```python
from build123d import *

# Parameters (mm, degrees)
F0_W     = 134.2057809234
F0_H     = 157.6057672501
F1_DEPTH = 25.4
F2_W     = 134.2057809234
F2_H     = 11.8888095021
F3_DEPTH = 50.8
F4_R     = 3.3067851736
F4_R_2   = 4.5017573087
F5_DEPTH = 25.4
F6_R     = 5.7930300282
F6_R_2   = 5.5883167401
F7_DEPTH = 25.4


with BuildPart() as f1:
    # F0 (on Front) → F1 (new body)
    with BuildSketch(Plane.XZ):
        with Locations((-1.6366653144, 9.6122771502)):
            Rectangle(F0_W, F0_H)
    extrude(amount=F1_DEPTH)

    # F2 (on face) → F3 (join)
    with BuildSketch(Plane.XZ.offset(25.4)):
        with Locations((-1.6366653144, -63.2462017238)):
            Rectangle(F2_W, F2_H)
    extrude(amount=F3_DEPTH)

    # F4 (on face) → F5 (cut)
    with BuildSketch(Plane.XY.offset(-57.3017969728)):
        with Locations((-55.1559180021, -38.2278487086)):
            Circle(F4_R)
        with Locations((-32.2959180021, -38.2278487086)):
            Circle(F4_R)
        with Locations((-9.4359180021, -38.2278487086)):
            Circle(F4_R)
        with Locations((13.4240819979, -38.2278487086)):
            Circle(F4_R)
        with Locations((36.2840819979, -38.2278487086)):
            Circle(F4_R)
        with Locations((59.1440819979, -38.2278487086)):
            Circle(F4_R)
        with Locations((-54.9669824541, -59.3341551721)):
            Circle(F4_R_2)
        with Locations((-29.5669824541, -59.3341551721)):
            Circle(F4_R_2)
        with Locations((-4.1669824541, -59.3341551721)):
            Circle(F4_R_2)
        with Locations((21.2330175459, -59.3341551721)):
            Circle(F4_R_2)
        with Locations((46.6330175459, -59.3341551721)):
            Circle(F4_R_2)
    extrude(amount=-F5_DEPTH, mode=Mode.SUBTRACT)

    # F6 (on face) → F7 (join)
    with BuildSketch(Plane.XZ.offset(25.4)):
        with Locations((-55.2074015141, 75.3232464194)):
            Circle(F6_R)
        with Locations((-33.8714015141, 75.3232464194)):
            Circle(F6_R)
        with Locations((-12.5354015141, 75.3232464194)):
            Circle(F6_R)
        with Locations((8.8005984859, 75.3232464194)):
            Circle(F6_R)
        with Locations((30.1365984859, 75.3232464194)):
            Circle(F6_R)
        with Locations((51.4725984859, 75.3232464194)):
            Circle(F6_R)
        with Locations((-57.3255419731, -8.0301519483)):
            Circle(F6_R_2)
        with Locations((-34.4655419731, -8.0301519483)):
            Circle(F6_R_2)
        with Locations((-11.6055419731, -8.0301519483)):
            Circle(F6_R_2)
        with Locations((11.2544580269, -8.0301519483)):
            Circle(F6_R_2)
        with Locations((34.1144580269, -8.0301519483)):
            Circle(F6_R_2)
        with Locations((56.9744580269, -8.0301519483)):
            Circle(F6_R_2)
    extrude(amount=F7_DEPTH)


solid = f1.part
```
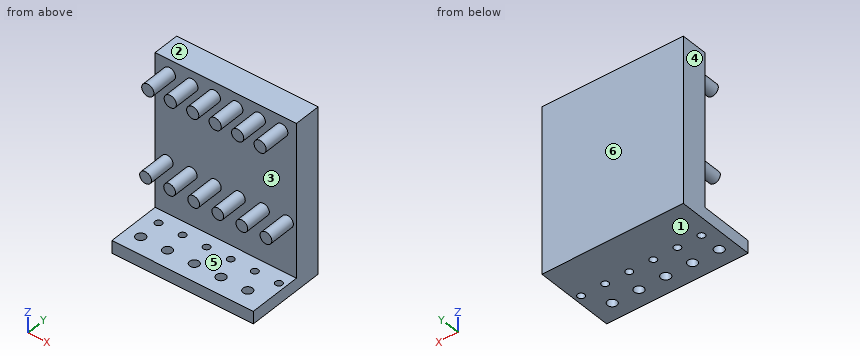
Here's how the part is built. I have some questions about the finished solid (model axes, mm). Face numbers are marked on the shaded views. A direction names the side the tool comes from. Coordinates: 2 decimals unless noted, no trailing zeros. Order: outer loops, then holes, each group sorted by start corner. A loop starts at its lowest first (then second) coordinate and runs counter-clockwise, first axis right, second up. Notation, with made-up numbers: (50, 65) - (63, 65) arc R12 ccw to (63, 74) - close; hole circle Ø9 at (45.25, -9). An arc over 180 degrees is marked (long way). One line per question, with ' | ' between items. Start each with the question number.
1. Please list where these lines run through material, in increasing order: line 1 along Z through (x, y) = (13.5, -44.5); line 2 along X through (y, z) = (-32, 72); line 3 along Z through (x, y) = (8, -34.5). Write a range as [from, to].
2. If we section it at D-D (x = -47): Write out the boundary of the cut face in (y, z), and give its area (3 significant figures).
3. I'm going to push flat-ended pins straight in: pin 1 Ø12.5 at (x, z) = (-58.5, -10.5) entering from -Y; pin 2 Ø8.5 at (x, y) = (36.28, -38.23) entering from +Z; pin 3 Ø6 at (x, y) = (13.42, -38.23) entering from +Z; pin 4 Ø7 at (x, y) = (-29.57, -59.33) entering from -Z. Where does each tip first touch, or does it pass through?
4. If we section it at B-B (x = -4): Write out the boundary of the cut face in (y, z), and give its area (3 significant figures).
5. If we section it at C-C (z = -5.5): Write out the boundary of the cut face in (x, y).
6. If we mould it in two halves opening along Z, with no side actions, what happens to the marked faces 1, 2, 3 and 4? For each: released by +Z, released by -Z, zero draft, split by the parting line, or undercut.
7. If we section it at A-A (y = -28): Give the number of separate pieces and of enclosed holes in the cut face, and give its area (3 significant figures).
8. Which directions (+Z, -Z, +X, -X, +Y, -Y) give clear straight access to the entire face, cutting with the end or side of a thin tool? Please do the marked faces 5 and 6.
Model answer:
1) line 1: z = [-69.19, -57.3], [-13.15, -2.91], [71.94, 78.71] | line 2: x = [-59.95, -50.46], [-38.62, -29.13], [-17.28, -7.79], [4.06, 13.55], [25.39, 34.88], [46.73, 56.22] | line 3: z = [-69.19, -57.3], [-12.57, -3.49], [69.59, 81.06]
2) outline: (-76.2, -69.19) - (0, -69.19) - (0, 88.42) - (-25.4, 88.42) - (-25.4, -57.3) - (-76.2, -57.3) - close | area: 4,610 mm²
3) pin 1: stops at y = -50.8 | pin 2: stops at z = 80.8 | pin 3: stops at z = 80.89 | pin 4: passes through
4) outline: (-76.2, -69.19) - (-63.83, -69.19) - (-63.83, -57.3) - (-76.2, -57.3) - close; (-54.84, -69.19) - (0, -69.19) - (0, 88.42) - (-25.4, 88.42) - (-25.4, -57.3) - (-54.84, -57.3) - close | area: 4,500 mm²
5) outline: (-68.74, -25.4) - (-62.31, -25.4) - (-62.31, -50.8) - (-52.34, -50.8) - (-52.34, -25.4) - (-39.45, -25.4) - (-39.45, -50.8) - (-29.48, -50.8) - (-29.48, -25.4) - (-16.59, -25.4) - (-16.59, -50.8) - (-6.62, -50.8) - (-6.62, -25.4) - (6.27, -25.4) - (6.27, -50.8) - (16.24, -50.8) - (16.24, -25.4) - (29.13, -25.4) - (29.13, -50.8) - (39.1, -50.8) - (39.1, -25.4) - (51.99, -25.4) - (51.99, -50.8) - (61.96, -50.8) - (61.96, -25.4) - (65.47, -25.4) - (65.47, 0) - (-68.74, 0) - close
6) face 1: released by -Z | face 2: released by +Z | face 3: undercut | face 4: zero draft
7) separate pieces: 13 | enclosed holes: 0 | area: 2,820 mm²
8) face 5: +X, -X, -Y | face 6: +Z, -Z, +X, -X, +Y
